Design review of the part built by this model. Coordinates are the model's own, in mm. A direction names the side the tool comes from. Round coordinates to 2 decimals unless told otherwise and drop trailing zeros. Loops run counter-clockwise (first coordinate to the right, second up) from the corner with the lowest first, then second, coordinate; pieces in that order, holes last. Notation, with made-up numbers: (64, 5) - (117, 5) arc R21 ccw to (117, 22) - close; hole circle Ø4 at (45.5, 39). An arc over 180 degrees is marked (long way). Use one line per item in the form item = value. Start each with the question number.
(1) We need section B-B, the plane z = -38. Write out the cut boundary in (x, y).
(2) We need section C-C, the plane z = 32.5. Write out the cut boundary in (x, y), then the cut area to 3 significant figures.
(3) For pin 1 (12 mm diameter, centred on x = -8, y = -36.5, fed in from -Z); pin 2 (6 mm diameter, centred on x = 11.5, z = 1, fed in from +Y); pin 3 (3 mm diameter, centred on y = 15, z = 16, fed in from -X); pin 4 (21 mm diameter, centred on y = 0, z = 0, fed in from +X), all flat-tipped, find the tip position at first contact; note any pin that passes through.
(4) Wall thickness on probe 1 along Y at (x, z) = (-20.1, 0); probe 2 along Y at (x, z) = (9.5, 2); probe 3 along Z at (x, y) = (3, 43.5): over which ranges is each line inside the solid? List them lowest first. Write a range as [from, to].
(5) Machinability: for faces 4 (the flat face through (0.31, -3.06, -46.02)), 5 (the cylindrical face through (-14.4, -39.23, -8.71)), 6 (the flat face through (0.308, 45.219, 9.623)), 7 (the flat face through (0.31, 31.86, -27.57)), which of the approach directions +Z, -Z, +X, -X, +Y, -Y give a long, thin tool a straight path to every point of the face, cutting with its end or side? Answer none if there is none.
(6) We need section A-A, the plane x = 13. Give the number of separate pieces and of enclosed holes in the cut face, then the cut area to 3 significant figures.
(7) The part is to be moulded in two halves that separate along Y. For faces 1 (the flat face through (0.308, -45.114, 9.577)), 2 (the flat face through (0.308, 46.098, -3.507)), 3 (the flat face through (0.3, -27.5, -37.1)), say which applies: released by +Y, released by -Y, zero draft, split by the parting line, or undercut.
from build123d import *

# Parameters (mm, degrees)
F3_DEPTH        = 48.6
F3_COPIES_COUNT = 22


# Not quite as in the source:
# - a pattern or mirror of a feature is missing from the dataset's text; its kind, count and spacing are read off the source's solid


with BuildPart() as f1:
    # F0 (on Front) → F1 (revolve)
    with BuildSketch(Plane.XZ):
        Polygon((22, 50.1841045916), (0, 50.1841045916), (-22, 50.1841045916), (-22, 40.1841045916), (-7, 40.1841045916), (-7, 16.1841045916), (-22, 16.1841045916), (-22, 9.1841045916), (-18, 9.1841045916), (-18, 11.1841045916), (-16, 11.1841045916), (-16, 9.1841045916), (-1.5, 9.1841045916), (-1.5, 7.1841045916), (0, 7.1841045916), (1.5, 7.1841045916), (1.5, 9.1841045916), (16, 9.1841045916), (16, 11.1841045916), (18, 11.1841045916), (18, 9.1841045916), (22, 9.1841045916), (22, 16.1841045916), (7, 16.1841045916), (7, 40.1841045916), (22, 40.1841045916), align=None)
    revolve(axis=Axis((-7.0416135713, 0, 0), (-1, 0, 0)))

    # F2 (on Right) → F3 (cut, symmetric)
    with BuildSketch(Plane.YZ):
        Polygon((-2, 42.1328544021), (0, 42.1328544021), (2, 42.1328544021), (5, 53.1328544021), (0, 53.1328544021), (-5, 53.1328544021), align=None)
    f3 = extrude(amount=F3_DEPTH, both=True, mode=Mode.SUBTRACT)

    # F3_copies: F3 ×22 about axis
    f3_copies_axis = Axis((0, 0, 0), (1, 0, 0))
    for i in range(1, F3_COPIES_COUNT):
        add(f3.rotate(f3_copies_axis, i * 360 / F3_COPIES_COUNT), mode=Mode.SUBTRACT)


solid = f1.part
Data:
q1.outline = (-22, -32.78) - (22, -32.78) - (22, -28.5) - (-22, -28.5) - close; (-22, -21.56) - (22, -21.56) - (22, -13.07) - (7, -13.07) - (7, 13.07) - (22, 13.07) - (22, 21.56) - (-22, 21.56) - (-22, 13.07) - (-7, 13.07) - (-7, -13.07) - (-22, -13.07) - close; (-22, 28.5) - (22, 28.5) - (22, 32.78) - (-22, 32.78) - close
q2.outline = (-22, -32.81) - (22, -32.81) - (22, -23.63) - (7, -23.63) - (7, 23.63) - (22, 23.63) - (22, 32.81) - (-22, 32.81) - (-22, 23.63) - (-7, 23.63) - (-7, -23.63) - (-22, -23.63) - close
q2.area = 1,470 mm^2
q3.pin_1 = -39.83
q3.pin_2 = 50.18
q3.pin_3 = -7
q3.pin_4 = 22
q4.probe_1 = [-50.18, -40.18], [-16.18, -9.18], [9.18, 16.18], [40.18, 50.18]
q4.probe_2 = [-50.14, -40.13], [-16.06, -8.96], [8.96, 16.06], [40.13, 50.14]
q4.probe_3 = [-25.02, -24.33], [-16.39, -8.88], [-3.83, 3.83], [8.88, 16.39], [24.33, 25.02]
q5.face_4 = -Z, +X, -X
q5.face_5 = -X
q5.face_6 = +X, -X, +Y
q5.face_7 = +X, -X
q6.separate_pieces = 2
q6.enclosed_holes = 2
q6.area = 2,310 mm^2
q7.face_1 = released by -Y
q7.face_2 = released by +Y
q7.face_3 = undercut
